The figure shows three views and two pictorial views of one solid part (mm, origin at its lowest corner). Answer the questions. A direction names the side the tool comes from. Coordinates: 2 decimals unless noted, no trailing zeros. Write each loop counter-clockwise with the first axis right and the second up, starting at its lowest first coordinate (ties: lowest second). Pieces come first, ordered by that corner, then holes.
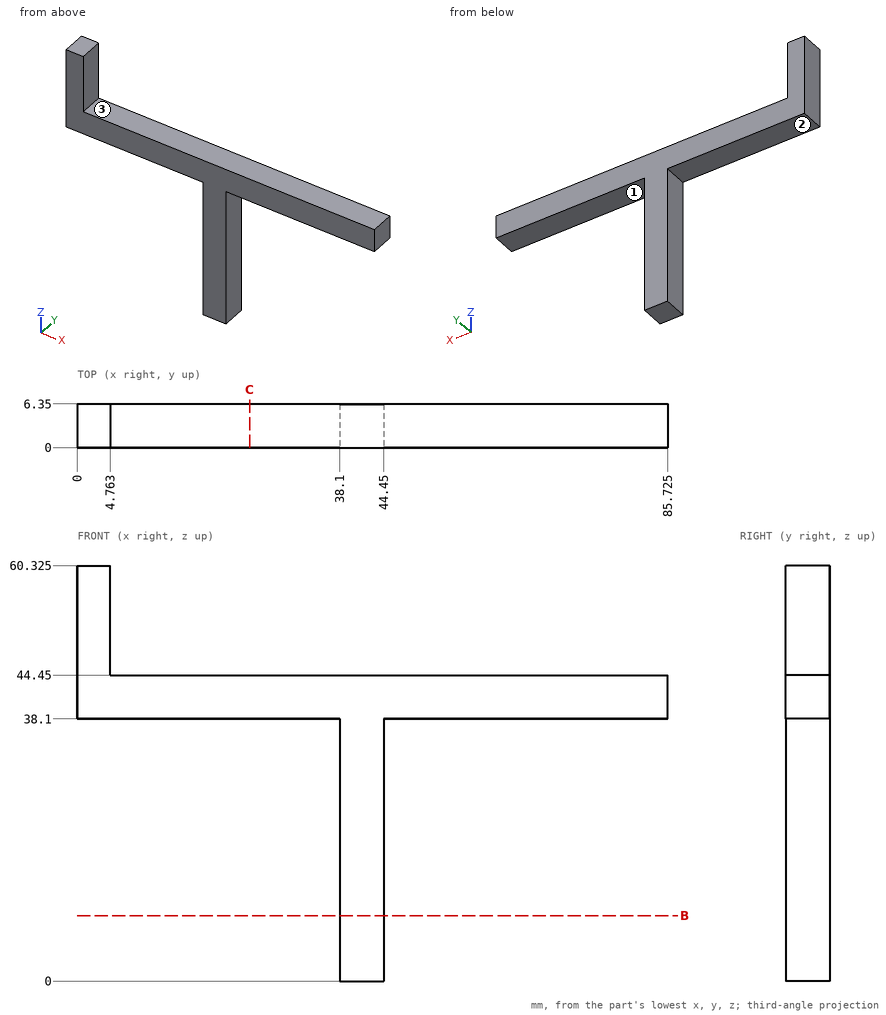
Item 1: The part is cut by section B-B (z = 9.5). Give the vertices of the cut face in (x, y).
Item 2: Given pin 1 (6 mm diameter, centred on x = 33.5, z = 20, fed in from -Y); pin 2 (1.9 mm diameter, centred on x = 28, y = 4.5, fed in from -Z), each flat-ended and moving along its own axis, determine where each tip first touches the part or whether it passes through.
Item 3: Find the intervals of material crossed by probe 1 along Z at (x, y) = (15.5, 5.5); probe 2 along X at (y, z) = (3.25, 44.5), in increasing order.
Item 4: For the marked faces 1, 2 and 3, determine the directions among +Z, -Z, +X, -X, +Y, -Y from which every point of the face is accessible in a straight line to the end or side of a thin tool.
Item 5: The part is cut by section C-C (x = 25). Give the vertices of the cut face in (y, z).
Answer:
1. outline: (38.1, 0) - (44.45, 0) - (44.45, 6.35) - (38.1, 6.35) - close
2. pin 1: passes through
2. pin 2: stops at z = 38.1
3. probe 1: z = 38.1 to 44.45
3. probe 2: x = 0 to 4.76
4. face 1: -Z, +X, +Y, -Y
4. face 2: -Z, -X, +Y, -Y
4. face 3: +Z, +X, +Y, -Y
5. outline: (0, 38.1) - (6.35, 38.1) - (6.35, 44.45) - (0, 44.45) - close
